```python
from build123d import *

# Parameters (mm, degrees)
SKETCH2_W                 = 95
SKETCH2_H                 = 96.52
BOSS_EXTRUDE3_DEPTH       = 5.08
SKETCH3_R                 = 22.225
CUT_EXTRUDE1_DEPTH        = 78.447905072
M6X1_0_TAPPED_HOLE1_D     = 5
M6X1_0_TAPPED_HOLE1_DEPTH = 5.08
M6X1_0_TAPPED_HOLE1_TIP   = 1.502151548
SKETCH7_R                 = 2.54
CUT_EXTRUDE2_DEPTH        = 7.62


with BuildPart() as part:
    # Sketch2 → Boss-Extrude3 (new body)
    with BuildSketch(Plane(origin=(0, 0, 0), x_dir=(1, 0, 0), z_dir=(0, 1, 0))):
        with Locations((0, -12.7)):
            Rectangle(SKETCH2_W, SKETCH2_H)
    extrude(amount=BOSS_EXTRUDE3_DEPTH)

    # Sketch3 → Cut-Extrude1 (cut, through all)
    with BuildSketch(Plane(origin=(0, 5.08, 0), x_dir=(1, 0, 0), z_dir=(0, 1, 0))):
        with Locations(Location((0, -21.59, 0), (0, 0, 270))):
            Circle(SKETCH3_R)
    extrude(amount=-CUT_EXTRUDE1_DEPTH, mode=Mode.SUBTRACT)

    # M6x1.0 Tapped Hole1
    with Locations(Plane(origin=(0, 5.08, 0), x_dir=(1, 0, 0), z_dir=(0, 1, 0))):
        with Locations((-40, 20.32), (40, 20.32), (0, 20.32)):
            Hole(M6X1_0_TAPPED_HOLE1_D / 2, depth=M6X1_0_TAPPED_HOLE1_DEPTH)
            with Locations((0, 0, -(M6X1_0_TAPPED_HOLE1_DEPTH + M6X1_0_TAPPED_HOLE1_TIP / 2))):  # 118° drill point
                Cone(0, M6X1_0_TAPPED_HOLE1_D / 2, M6X1_0_TAPPED_HOLE1_TIP, mode=Mode.SUBTRACT)

    # Sketch7 → Cut-Extrude2 (cut)
    with BuildSketch(Plane(origin=(0, 5.08, 0), x_dir=(1, 0, 0), z_dir=(0, 1, 0))):
        with Locations(Location((-33.02, -44.45, 0), (0, 0, 270))):
            Circle(SKETCH7_R)
        with Locations(Location((33.02, -44.45, 0), (0, 0, 270))):
            Circle(SKETCH7_R)
        with Locations(Location((-38.1, -52.07, 0), (0, 0, 270))):
            Circle(SKETCH7_R)
        with Locations(Location((38.1, -52.07, 0), (0, 0, 270))):
            Circle(SKETCH7_R)
    extrude(amount=-CUT_EXTRUDE2_DEPTH, mode=Mode.SUBTRACT)


solid = part.part
```
Verification items for the finished model (mm, model axes). Coordinates: 2 decimals unless noted, no trailing zeros. Loops run counter-clockwise (first coordinate to the right, second up) from the corner with the lowest first, then second, coordinate; pieces in that order, holes last. Notation, with made-up numbers: (30.5, -6) - (72.5, -6) arc R13 cw to (72.5, 17) - close; hole circle Ø9 at (-30.5, 2.25). An arc over 180 degrees is marked (long way). Put each result on its own line as item: value.
Item 1: Draft check along Z on faces 1 (the face through (47.5, 3, 13)), 2 (the face through (-1, 3, -35.56)), 3 (the face through (37.615, 2.504, -21.071)). Enter one of: pulls with the +Z half, pulls with the -Z half, needs draft (parallel to the pull), parting line crosses it, or undercut.
Conclusion:
face 1: needs draft
face 2: pulls with the -Z half
face 3: undercut
Item 2: Section check D-D (z = -20.32). Enter the section's corners in (x, y).
Conclusion:
outline: (-47.5, 0) - (-42.5, 0) - (-42.5, 5.08) - (-47.5, 5.08) - close; (-37.5, 0) - (-2.5, 0) - (-2.5, 5.08) - (-37.5, 5.08) - close; (2.5, 0) - (37.5, 0) - (37.5, 5.08) - (2.5, 5.08) - close; (42.5, 0) - (47.5, 0) - (47.5, 5.08) - (42.5, 5.08) - close
Item 3: Section check A-A (z = 21.59). Enter the section's corners in (x, y) (3 decimals).
Conclusion:
outline: (-47.5, 0) - (-22.225, 0) - (-22.225, 5.08) - (-47.5, 5.08) - close; (22.225, 0) - (47.5, 0) - (47.5, 5.08) - (22.225, 5.08) - close
Item 4: Section check C-C (x = -33.02). Enter the section's corners in (y, z).
Conclusion:
outline: (0, -35.56) - (5.08, -35.56) - (5.08, 41.91) - (0, 41.91) - close; (0, 46.99) - (5.08, 46.99) - (5.08, 60.96) - (0, 60.96) - close
Item 5: Scan lines: line 1 along X through (y, z) = (2.65, 44.45); line 2 along X through (y, z) = (1.2, 52.07); line 3 along X through (y, z) = (3.4, -20.32). Record each from-to range of solid material in increasing order.
Conclusion:
line 1: x = -47.5 to -35.56, -30.48 to 30.48, 35.56 to 47.5
line 2: x = -47.5 to -40.64, -35.56 to 35.56, 40.64 to 47.5
line 3: x = -47.5 to -42.5, -37.5 to -2.5, 2.5 to 37.5, 42.5 to 47.5
Item 6: Section check B-B (y = 4.25). Give the number of separate pieces and of enclosed holes in the cut face, then the cut area to 3 significant figures.
Conclusion:
separate pieces: 1
enclosed holes: 8
area: 7,480 mm2
